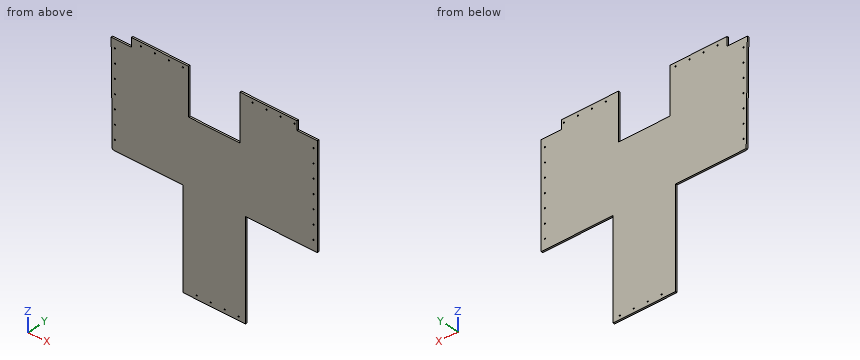
```python
from build123d import *

# Parameters (mm, degrees)
BOSS_EXTRUDE1_DEPTH = 5
SKETCH2_R           = 1.75
CUT_EXTRUDE1_DEPTH  = 6


with BuildPart() as part:
    # Sketch1 → Boss-Extrude1 (new body)
    with BuildSketch(Plane(origin=(0, 329.925662842, 0), x_dir=(1, 0, 0), z_dir=(0, 1, 0))):
        Polygon((180.899872759, -210.782719675), (180.899872759, 70.717280325), (359.699872759, 70.717280325), (359.699872759, -210.782719675), (565.699872759, -210.782719675), (565.699872759, -503.882719675), (507.724872759, -503.882719675), (507.724872759, -529.282719675), (344.299872759, -529.282719675), (344.299872759, -396.017719675), (196.299872759, -396.017719675), (196.299872759, -529.282719675), (32.874872759, -529.282719675), (32.874872759, -503.882719675), (-25.100127241, -503.882719675), (-21.925127241, -210.782719675), align=None)
    extrude(amount=BOSS_EXTRUDE1_DEPTH)

    # Sketch2 → Cut-Extrude1 (cut, through all)
    with BuildSketch(Plane.XZ.offset(-329.925662842)):
        with Locations((60.299872759, 518.607719675)):
            Circle(SKETCH2_R)
        with Locations((380.299872759, 518.607719675)):
            Circle(SKETCH2_R)
        with Locations((220.299872759, -60.042280325)):
            Circle(SKETCH2_R)
        with Locations((100.299872759, 518.607719675)):
            Circle(SKETCH2_R)
        with Locations((420.299872759, 518.607719675)):
            Circle(SKETCH2_R)
        with Locations((260.299872759, -60.042280325)):
            Circle(SKETCH2_R)
        with Locations((140.299872759, 518.607719675)):
            Circle(SKETCH2_R)
        with Locations((460.299872759, 518.607719675)):
            Circle(SKETCH2_R)
        with Locations((300.299872759, -60.042280325)):
            Circle(SKETCH2_R)
        with Locations((180.299872759, 518.607719675)):
            Circle(SKETCH2_R)
        with Locations((500.299872759, 518.607719675)):
            Circle(SKETCH2_R)
        with Locations((340.299872759, -60.042280325)):
            Circle(SKETCH2_R)
        with Locations((-14.425127241, 239.282719675)):
            Circle(SKETCH2_R)
        with Locations((555.024872759, 239.282719675)):
            Circle(SKETCH2_R)
        with Locations((-14.425127241, 279.282719675)):
            Circle(SKETCH2_R)
        with Locations((555.024872759, 279.282719675)):
            Circle(SKETCH2_R)
        with Locations((-14.425127241, 319.282719675)):
            Circle(SKETCH2_R)
        with Locations((555.024872759, 319.282719675)):
            Circle(SKETCH2_R)
        with Locations((-14.425127241, 359.282719675)):
            Circle(SKETCH2_R)
        with Locations((555.024872759, 359.282719675)):
            Circle(SKETCH2_R)
        with Locations((-14.425127241, 399.282719675)):
            Circle(SKETCH2_R)
        with Locations((555.024872759, 399.282719675)):
            Circle(SKETCH2_R)
        with Locations((-14.425127241, 439.282719675)):
            Circle(SKETCH2_R)
        with Locations((555.024872759, 439.282719675)):
            Circle(SKETCH2_R)
        with Locations((-14.425127241, 479.282719675)):
            Circle(SKETCH2_R)
        with Locations((555.024872759, 479.282719675)):
            Circle(SKETCH2_R)
    extrude(amount=-CUT_EXTRUDE1_DEPTH, mode=Mode.SUBTRACT)


solid = part.part
```
CAD build for the part. Positions are in the model's coordinates, mm. Round coordinates to 2 decimals unless told otherwise and drop trailing zeros. Order: outer loops, then holes, each group sorted by start corner. A loop starts at its lowest first (then second) coordinate and runs counter-clockwise, first axis right, second up. Notation, with made-up numbers: (47.5, 34.5) - (75.5, 34.5) arc R26 cw to (75.5, 63.5) - close; hole circle Ø4 at (89, 77). An arc over 180 degrees is marked (long way). Use CSV: the item, a comma, the result in double quotes. Start each with the question number.
1) Saw through at B-B (x = 290.5). List the corners of the cut face in (y, z).
2) Pin check, flat tips, straight feed: pin 1 Ø5.5 at (x, z) = (-14.43, 319.28) entering from -Y; pin 2 Ø2.5 at (y, z) = (331.5, 512) entering from +X. Stop position of each tip, or through.
3) Saw through at D-D (y = 332.9). Count the separate pieces of the cut face and the enclosed holes in it, and give its area (3 significant figures).
4) Saw through at C-C (z = 151). List the corners of the cut face in (x, y), and give its area (3 significant figures).
5) Saw through at A-A (z = 456). List the corners of the cut face in (x, y), and give its area (3 significant figures).
6) Wall check: L1, parallel to X at y = 333.4, z = 501; L2, parallel to X at y = 333.75, z = 201; L3, parallel to Z at x = 383.5, y = 332.5. Give the ranges that are in metal, low to high. Write a range as [from, to].
Values follow:
1,outline,"(329.93, -70.72) - (334.93, -70.72) - (334.93, 396.02) - (329.93, 396.02) - close"
2,pin 1,"stops at y = 329.93"
2,pin 2,"stops at x = 507.72"
3,separate pieces,"1"
3,enclosed holes,"26"
3,area,"215,000 mm2"
4,outline,"(180.9, 329.93) - (359.7, 329.93) - (359.7, 334.93) - (180.9, 334.93) - close"
4,area,"894 mm2"
5,outline,"(-24.58, 329.93) - (196.3, 329.93) - (196.3, 334.93) - (-24.58, 334.93) - close; (344.3, 329.93) - (565.7, 329.93) - (565.7, 334.93) - (344.3, 334.93) - close"
5,area,"2,210 mm2"
6,L1,"x = [-25.07, 196.3], [344.3, 565.7]"
6,L2,"x = [180.9, 359.7]"
6,L3,"z = [210.78, 529.28]"
